Read the model definition and answer for the solid it produces. Units are mm, in the model's axes. A direction names the side the tool comes from. Round coordinates to 2 decimals unless told otherwise and drop trailing zeros. Loops run counter-clockwise (first coordinate to the right, second up) from the corner with the lowest first, then second, coordinate; pieces in that order, holes last. Notation, with made-up numbers: (58, 86.5) - (103, 86.5) arc R14 ccw to (103, 99.5) - close; hole circle Ø5 at (3.25, 83.25). An arc over 180 degrees is marked (long way). Use CSV: the item, a comma, the result in double quotes. Start each with the question number.
1. Find section C-C (z = -1). Give the vertices of the cut face in (x, y), and give its area (3 significant figures).
2. Find section A-A (x = -0.45). Give the vertices of the cut face in (y, z).
3. Find section D-D (y = 8). Give the vertices of the cut face in (x, z).
4. A tool of negligible diameter and unlimited length cuts with its end or side. For faces 1 (the flat face through (0, 1, -2)), 2 (the flat face through (-1, 2.25, -2)), 3 (the flat face through (-3.536, 5, -6)), from which of +Z, -Z, +X, -X, +Y, -Y can it reach the whole face along a straight path? Write none if from no direction.
5. Consider line 1 along Y through (x, z) = (-0.6, -2.25); line 2 along X through (y, z) = (5.75, 0); line 3 along X through (y, z) = (5.25, -4.5). Determine where each line is inside the solid, lowest interval first.
6. Given pin 1 Ø0.7 at (y, z) = (4, -6) entering from -X, flat-ended and moving along its own axis, determine where the tip first touches the part or whether it passes through.
7. Determine the mould class of faces 4 (the flat face through (-1.51, 6.661, 0.252)), 5 (the flat face through (-2, 10, -2)), 6 (the flat face through (-3.536, 5, 2)) for opening direction Y: +Y half, -Y half, draft (parallel to the pull), parting line (faces both ways), or undercut.
8. Find section B-B (y = 4.5). Give the vertices of the cut face in (x, z), and give its area (3 significant figures).
Autodesk Inventor part; units mm, degrees
ref_plane "YZ Plane" through (0, 0, 0) normal (1, 0, 0) x (0, 1, 0)
ref_plane "XZ Plane" through (0, 0, 0) normal (0, 1, 0) x (-1, 0, 0)
ref_plane "XY Plane" through (0, 0, 0) normal (0, 0, 1) x (1, 0, 0)
sketch "Sketch1" plane through (0, 0, 0) normal (0, 1, 0) x (-1, 0, 0)
  line L0 (0, 0) -> (3.5355, 3.5355)
  line L1 (3.5355, 3.5355) -> (3.5355, 0.0355)
  line L2 (3.5355, 0.0355) -> (5.0355, 1.5355)
  line L3 (5.0355, 1.5355) -> (5.0355, -5.4645)
  line L4 (5.0355, -5.4645) -> (3.5355, -3.9645)
  line L5 (3.5355, -3.9645) -> (3.5355, -7.4645)
  line L6 (3.5355, -7.4645) -> (0, -3.929)
  line L7 (0, -3.929) -> (0, 0)
  dimension "d0" = 3.929
  dimension "d1" = 5
  dimension "d2" = 5
  dimension "d3" = 3.5
  dimension "d4" = 3.5
  dimension "d5" = 135
  dimension "d6" = 45
  dimension "d7" = 1.5
extrude "Extrusion1" add sketch "Sketch1" along normal blind 10
fillet "Fillet1" radius 0.25 6 edges at (-3.5355, 5, -3.9645) (-3.5355, 5, -7.4645) (-5.0355, 5, -5.4645) (-3.5355, 5, 3.5355) (-3.5355, 5, 0.0355) (-5.0355, 5, 1.5355)
sketch "Sketch2" plane through (0, 0, 0) normal (1, 0, 0) x (0, 0, -1)
  line L0 (0.3768, 7.75) -> (3.5522, 7.75)
  line L1 (3.5522, 7.75) -> (5.1399, 5)
  line L2 (5.1399, 5) -> (3.5522, 2.25)
  line L3 (3.5522, 2.25) -> (0.3768, 2.25)
  line L4 (0.3768, 2.25) -> (-1.2109, 5)
  line L5 (-1.2109, 5) -> (0.3768, 7.75)
  line L6 (3.929, 0) -> (3.929, 10)
  line L7 (0, 10) -> (3.929, 10)
  point P0 (0, 0)
  point P1 (1.9645, 5)
  dimension "d11" = 5.5
  dimension "d12" = 1.9645
  dimension "d13" = 5
extrude "Extrusion2" cut sketch "Sketch2" against normal blind 2.5
sketch "Sketch3" plane through (-2.5, 0, 0) normal (1, 0, 0) x (0, 0, -1)
  circle A0 centre (1.9645, 5) radius 1.6
  line L0 (3.929, 0) -> (3.929, 2.9026)
  line L1 (0, 10) -> (3.929, 10)
  point P0 (0, 0)
  dimension "d16" = 3.2
  dimension "d17" = 1.9645
  dimension "d18" = 5
extrude "Extrusion3" cut sketch "Sketch3" against normal through all
properties part number "nut"
Filled sheet:
1,outline,"(-5.04, 0) - (0, 0) - (0, 2.25) - (-2.5, 2.25) - (-2.5, 3.72) - (-5.04, 3.72) - close; (-5.04, 6.28) - (-2.5, 6.28) - (-2.5, 7.75) - (0, 7.75) - (0, 10) - (-5.04, 10) - close"
1,area,"30.1 mm²"
2,outline,"(0, -4.38) - (3.68, -4.38) - (2.25, -3.55) - (2.25, -0.38) - (3.68, 0.45) - (0, 0.45) - close; (6.32, -4.38) - (10, -4.38) - (10, 0.45) - (6.32, 0.45) - (7.75, -0.38) - (7.75, -3.55) - close"
3,outline,"(-5.04, -4.86) arc R0.25 ccw to (-4.61, -5.04) - (-3.96, -4.39) arc R0.25 cw to (-3.54, -4.57) - (-3.54, -6.86) arc R0.25 ccw to (-3.11, -7.04) - (0, -3.93) - (0, 0) - (-3.11, 3.11) arc R0.25 ccw to (-3.54, 2.93) - (-3.54, 0.64) arc R0.25 cw to (-3.96, 0.46) - (-4.61, 1.11) arc R0.25 ccw to (-5.04, 0.93) - close"
4,face 1,"+Z, -Z, +X, +Y, -Y"
4,face 2,"+X"
4,face 3,"-Z, +Y, -Y"
5,line 1,"y = 0 to 2.25, 7.75 to 10"
5,line 2,"x = -5.04 to -2.5"
5,line 3,"x = -5.04 to -4.07, -3.54 to -2.5"
6,pin 1,"stops at x = -3.54"
7,face 4,"undercut"
7,face 5,"+Y half"
7,face 6,"draft"
8,outline,"(-5.04, -4.86) arc R0.25 ccw to (-4.61, -5.04) - (-3.96, -4.39) arc R0.25 cw to (-3.54, -4.57) - (-3.54, -6.86) arc R0.25 ccw to (-3.11, -7.04) - (-0.92, -4.85) - (-2.5, -4.85) - (-2.5, -3.48) - (-5.04, -3.48) - close; (-5.04, -0.44) - (-2.5, -0.44) - (-2.5, 0.92) - (-0.92, 0.92) - (-3.11, 3.11) arc R0.25 ccw to (-3.54, 2.93) - (-3.54, 0.64) arc R0.25 cw to (-3.96, 0.46) - (-4.61, 1.11) arc R0.25 ccw to (-5.04, 0.93) - close"
8,area,"13.2 mm²"
